from build123d import *

# Parameters (mm, degrees)
SKETCH2_W           = 24.765
SKETCH2_H           = 17.4625
BOSS_EXTRUDE1_DEPTH = 19.05
SKETCH3_W           = 28.575
SKETCH3_H           = 22.86
BOSS_EXTRUDE2_DEPTH = 38.1
SKETCH4_W           = 6.35
SKETCH4_H           = 23.8125
SKETCH4_W_2         = 11.049
CUT_EXTRUDE1_DEPTH  = 47.6725
SKETCH5_W           = 19.05
SKETCH5_H           = 8.89
BOSS_EXTRUDE3_DEPTH = 19.05
FILLET1_R           = 9.525
SKETCH6_R           = 4.7625
CUT_EXTRUDE2_DEPTH  = 50.382672553
FILLET5_R           = 11.43
SKETCH7_R           = 6.604
CUT_EXTRUDE3_DEPTH  = 54.615212627
FILLET2_R           = 2.54
FILLET3_R           = 6.35
FILLET6_R           = 1.27


# Some blends are built 0.0001 mm under size
with BuildPart() as part:
    # Sketch2 → Boss-Extrude1 (new body)
    with BuildSketch(Plane.XY):
        Rectangle(SKETCH2_W, SKETCH2_H)
    extrude(amount=-BOSS_EXTRUDE1_DEPTH)

    # Sketch3 → Boss-Extrude2 (add)
    with BuildSketch(Plane.XY):
        Rectangle(SKETCH3_W, SKETCH3_H)
    extrude(amount=BOSS_EXTRUDE2_DEPTH)

    # Sketch4 → Cut-Extrude1 (cut, through all)
    with BuildSketch(Plane(origin=(0, -11.43, 0), x_dir=(-1, 0, 0), z_dir=(0, -1, 0))):
        with Locations((11.1125, -26.19375)):
            Rectangle(SKETCH4_W, SKETCH4_H)
        with Locations((-3.175, -26.19375)):
            Rectangle(SKETCH4_W_2, SKETCH4_H)
    extrude(amount=-CUT_EXTRUDE1_DEPTH, mode=Mode.SUBTRACT)

    # Sketch5 → Boss-Extrude3 (add)
    with BuildSketch(Plane.XZ.offset(11.43)):
        with Locations((0, 6.4135)):
            Rectangle(SKETCH5_W, SKETCH5_H)
    extrude(amount=BOSS_EXTRUDE3_DEPTH)

    # Fillet1
    fillet1_edges = [part.edges().sort_by_distance(p)[0] for p in [
        (9.525, -30.48, 6.4135),
        (-9.525, -30.48, 6.4135),
    ]]
    fillet(fillet1_edges, radius=FILLET1_R - 0.0001)  # a hair under: the kernel refuses the full size

    # Sketch6 → Cut-Extrude2 (cut, through all)
    with BuildSketch(Plane(origin=(0, 0, 1.9685), x_dir=(-1, 0, 0), z_dir=(0, 0, -1))):
        with Locations((0, -20.955)):
            Circle(SKETCH6_R)
    extrude(amount=-CUT_EXTRUDE2_DEPTH, mode=Mode.SUBTRACT)

    # Fillet5
    fillet5_edges = [part.edges().sort_by_distance(p)[0] for p in [
        (-5.1435, -11.43, 38.1),
        (-5.1435, 11.43, 38.1),
        (11.4935, 11.43, 38.1),
        (11.4935, -11.43, 38.1),
    ]]
    fillet(fillet5_edges, radius=FILLET5_R - 0.0001)  # a hair under: the kernel refuses the full size

    # Sketch7 → Cut-Extrude3 (cut, through all)
    with BuildSketch(Plane.ZY.offset(7.9375)):
        with Locations(Location((26.67, 0, 0), (0, 0, 270))):
            Circle(SKETCH7_R)
    extrude(amount=-CUT_EXTRUDE3_DEPTH, mode=Mode.SUBTRACT)

    # Fillet2
    # the kernel refuses this fillet: 2.54 mm, written as the material it takes off along each edge
    with BuildSketch(Plane(origin=(-9.525, -11.43, 10.8585), x_dir=(0, 0, -1), z_dir=(0, -1, 0))) as fillet2_piece_1:
        with BuildLine():
            CenterArc((FILLET2_R, FILLET2_R), FILLET2_R, 180, 90)
            Line((0, FILLET2_R), (0, 0))
            Line((0, 0), (FILLET2_R, 0))
        make_face()
    extrude(amount=9.5251, mode=Mode.SUBTRACT)
    with BuildSketch(Plane(origin=(9.525, -11.43, 10.8585), x_dir=(0, 0, -1), z_dir=(0, -1, 0)), Plane(origin=(9.525, -11.43, 1.9685), x_dir=(-1, 0, 0), z_dir=(0, -1, 0)), Plane(origin=(-9.525, -11.43, 1.9685), x_dir=(0, 0, 1), z_dir=(0, -1, 0))) as fillet2_piece_2:
        with BuildLine():
            CenterArc((FILLET2_R, -FILLET2_R), FILLET2_R, 90, 90)
            Line((0, -FILLET2_R), (0, 0))
            Line((0, 0), (FILLET2_R, 0))
        make_face()
    extrude(amount=9.5251, mode=Mode.SUBTRACT)
    with BuildSketch(Plane(origin=(-0.0001, -20.9551, 10.8585), x_dir=(-1, 0, 0), z_dir=(0, 1, 0))) as fillet2_piece_3:
        with BuildLine():
            CenterArc((9.5249 - FILLET2_R, -FILLET2_R), FILLET2_R, 360, 90)
            Line((9.5249, -FILLET2_R), (9.5249, 0))
            Line((9.5249, 0), (9.5249 - FILLET2_R, 0))
        make_face()
    revolve(axis=Axis((-0.0001, -20.9551, 10.8585), (0, 0, 1)), revolution_arc=90, mode=Mode.SUBTRACT)
    with BuildSketch(Plane(origin=(0.0001, -20.9551, 10.8585), x_dir=(1, 0, 0), z_dir=(0, 1, 0))) as fillet2_piece_4:
        with BuildLine():
            CenterArc((9.5249 - FILLET2_R, FILLET2_R), FILLET2_R, 270, 90)
            Line((9.5249, FILLET2_R), (9.5249, 0))
            Line((9.5249, 0), (9.5249 - FILLET2_R, 0))
        make_face()
    revolve(axis=Axis((0.0001, -20.9551, 10.8585), (0, 0, -1)), revolution_arc=90, mode=Mode.SUBTRACT)
    with BuildSketch(Plane(origin=(-0.0001, -20.9551, 1.9685), x_dir=(-1, 0, 0), z_dir=(0, 1, 0))) as fillet2_piece_5:
        with BuildLine():
            CenterArc((9.5249 - FILLET2_R, FILLET2_R), FILLET2_R, 270, 90)
            Line((9.5249, FILLET2_R), (9.5249, 0))
            Line((9.5249, 0), (9.5249 - FILLET2_R, 0))
        make_face()
    revolve(axis=Axis((-0.0001, -20.9551, 1.9685), (0, 0, 1)), revolution_arc=90, mode=Mode.SUBTRACT)
    with BuildSketch(Plane(origin=(0.0001, -20.9551, 1.9685), x_dir=(1, 0, 0), z_dir=(0, 1, 0))) as fillet2_piece_6:
        with BuildLine():
            CenterArc((9.5249 - FILLET2_R, -FILLET2_R), FILLET2_R, 0, 90)
            Line((9.5249, -FILLET2_R), (9.5249, 0))
            Line((9.5249, 0), (9.5249 - FILLET2_R, 0))
        make_face()
    revolve(axis=Axis((0.0001, -20.9551, 1.9685), (0, 0, -1)), revolution_arc=90, mode=Mode.SUBTRACT)
    with BuildSketch(Plane(origin=(0, -20.955, 10.8585), x_dir=(-1, 0, 0), z_dir=(0, -1, 0))) as fillet2_piece_7:
        with BuildLine():
            CenterArc((4.7625 + FILLET2_R, FILLET2_R), FILLET2_R, 180, 90)
            Line((4.7625, FILLET2_R), (4.7625, 0))
            Line((4.7625, 0), (4.7625 + FILLET2_R, 0))
        make_face()
    revolve(axis=Axis((0, -20.955, 10.8585), (0, 0, -1)), mode=Mode.SUBTRACT)
    with BuildSketch(Plane(origin=(0, -20.955, 1.9685), x_dir=(-1, 0, 0), z_dir=(0, -1, 0))) as fillet2_piece_8:
        with BuildLine():
            CenterArc((4.7625 + FILLET2_R, -FILLET2_R), FILLET2_R, 90, 90)
            Line((4.7625, -FILLET2_R), (4.7625, 0))
            Line((4.7625, 0), (4.7625 + FILLET2_R, 0))
        make_face()
    revolve(axis=Axis((0, -20.955, 1.9685), (0, 0, -1)), mode=Mode.SUBTRACT)
    with BuildSketch(Plane(origin=(0.0001, -30.48, 1.9685), x_dir=(0, 1, 0), z_dir=(-1, 0, 0)), Plane(origin=(-0.0001, -30.48, 10.8585), x_dir=(0, 1, 0), z_dir=(1, 0, 0))) as fillet2_piece_9:
        with BuildLine():
            CenterArc((FILLET2_R, -FILLET2_R), FILLET2_R, 90, 90)
            Line((0, -FILLET2_R), (0, 0))
            Line((0, 0), (FILLET2_R, 0))
        make_face()
    extrude(amount=0.0002, mode=Mode.SUBTRACT)

    # Fillet3
    fillet3_edges = [part.edges().sort_by_distance(p)[0] for p in [
        (-12.3825, 8.73125, -9.525),
        (12.3825, 8.73125, -9.525),
        (12.3825, -8.73125, -9.525),
        (-12.3825, -8.73125, -9.525),
    ]]
    fillet(fillet3_edges, radius=FILLET3_R)

    # Fillet6
    fillet6_edges = [part.edges().sort_by_distance(p)[0] for p in [
        (-11.1125, -11.43, 14.2875),
        (3.175, -11.43, 14.2875),
    ]]
    fillet(fillet6_edges, radius=FILLET6_R)


solid = part.part
Source: CAD feature listing. Evaluate the final solid. Frame: model axes, mm. A direction names the side the tool comes from. Give positions to 0.01 mm unless a question says otherwise; leave off trailing zeros. Write each loop counter-clockwise with the first axis right and the second up, starting at its lowest first coordinate (ties: lowest second). Pieces come first, ordered by that corner, then holes. Notation, with made-up numbers: M 76.25,-20 L 80.25,-20 A32 ccw 80.25,6 Z; hole C -24,31.5 d9. An arc over 180 degrees is marked long. Return JSON: item names as keys, results as strings. Group by question number.
1) Material intervals for line 1 along Z through (x, y) = (-5.1, 0); line 2 along X through (y, z) = (8.5, 28); line 3 along X through (y, z) = (-22.5, 6.5), sorted ascending. Write a range as [from, to].
2) Pull-direction query (Y, two-part tool) for faces 1 (the face through (8.7, 2, 20)), 2 (the face through (-5.183, 0.86, 33.218)), 3 (the face through (3.098, -11.068, 13.906)); classes: pulls with the +Y half, pulls with the -Y half, needs draft (parallel to the pull), parting line crosses it, or undercut.
3) Set-up query: faces 4 (the face through (3, 0, 14.288)), 5 (the face through (0, 10, 0)), 6 (the face through (12.382, 0, -9)), 7 (the face through (8.801, -16.126, 10.095)), 8 (the face through (0, -13, 1.968)). Return all of +Z, -Z, +X, -X, +Y, -Y with unobstructed straight access to the full face (end or side cutting, diameter ignored); none if empty.
4) Cut plane A-A, the plane z = 31. Output: boundary loops of the cut face in (x, y).
5) Pin query (flat end, axial travel): P1, Ø1, axis at x = 0.5, y = -11, coming from the -Z side; P2, Ø5, axis at y = 0.5, z = -14, coming from the +X side; P3, Ø8, axis at x = 2.5, y = -16, coming from the +Z side. Return the tip coordinate at first contact, or that it passes through.
6) Cut plane B-B, the plane x = -10.75. Output: boundary loops of the cut face in (y, z).
Recorded:
{
 "1": {"line 1": "z = [-19.05, 20.07], [33.27, 38.1]", "line 2": "x = [-7.94, -2.35], [8.7, 14.29]", "line 3": "x = [-9.4, -4.5], [4.5, 9.4]"},
 "2": {"face 1": "needs draft", "face 2": "undercut", "face 3": "pulls with the -Y half"},
 "3": {"face 4": "+Z, +Y, -Y", "face 5": "-Z", "face 6": "-Z, +X, +Y, -Y", "face 7": "+Z, +X, -Y", "face 8": "-Z, +X, -X, -Y"},
 "4": {"outline": "M -7.94,-10.58 L -2.35,-10.58 L -2.35,-4.99 L -7.94,-4.99 Z; M -7.94,4.99 L -2.35,4.99 L -2.35,10.58 L -7.94,10.58 Z; M 8.7,-10.58 L 14.29,-10.58 L 14.29,-4.99 L 8.7,-4.99 Z; M 8.7,4.99 L 14.29,4.99 L 14.29,10.58 L 8.7,10.58 Z"},
 "5": {"P1": "stops at z = 0", "P2": "stops at x = 12.38", "P3": "stops at z = 10.86"},
 "6": {"outline": "M -11.43,0 L -6.63,0 L -6.63,-19.05 L 6.63,-19.05 L 6.63,0 L 11.43,0 L 11.43,14.29 L -10.16,14.29 A1.27 ccw -11.43,13.02 Z"}
}
